```python
from build123d import *

# Parameters (mm, degrees)
SKETCH_1_W      = 200
SKETCH_1_H      = 200
SKETCH_1_R      = 5
EXTRUDE_1_DEPTH = 5
CHAMFER_1_SIZE  = 3


with BuildPart() as part:
    # Эскиз1 → Бобышка-Вытянуть1 (new body)
    with BuildSketch(Plane(origin=(0, 0, 0), x_dir=(1, 0, 0), z_dir=(0, 1, 0))):
        Rectangle(SKETCH_1_W, SKETCH_1_H)
        Circle(SKETCH_1_R, mode=Mode.SUBTRACT)
    extrude(amount=EXTRUDE_1_DEPTH)

    # Фаска1
    chamfer_1_edges = [part.edges().sort_by_distance(p)[0] for p in [
        (-5, 0, 0),
    ]]
    chamfer(chamfer_1_edges, length=CHAMFER_1_SIZE)


solid = part.part
```
Input: part model. Units: mm. Frame: model coordinates. Coordinates: 2 decimals unless noted, no trailing zeros. Loops run counter-clockwise (first coordinate to the right, second up) from the corner with the lowest first, then second, coordinate; pieces in that order, holes last. Notation, with made-up numbers: (70, -12) - (108, -12) arc R30 cw to (108, 15) - close; hole circle Ø2 at (-30.5, 3.5). An arc over 180 degrees is marked (long way). Answer in a Markdown table with one row per item.
(1) Mould query, pull axis X, two halves, no side actions, for faces 1 (the face through (4.95, 2.81, -1.56)), 2 (the face through (-1, 0, -24)), 3 (the face through (100, 2, 1)). Classes: pulls with the +X half, pulls with the -X half, needs draft (parallel to the pull), parting line crosses it, or undercut.
Model answer:
| item | result |
|---|---|
| face 1 | undercut |
| face 2 | needs draft |
| face 3 | pulls with the +X half |
(2) Material intervals for L1, parallel to X at y = 4.45, z = 0, sorted ascending. Write a range as from..to.
Model answer:
| item | result |
|---|---|
| L1 | x = -100..-5, 5..100 |
(3) Cut plane B-B on z = 0. Output: boundary loops of the cut face in (x, y).
Model answer:
| item | result |
|---|---|
| outline | (-100, 0) - (-8, 0) - (-5, 3) - (-5, 5) - (-100, 5) - close; (5, 3) - (8, 0) - (100, 0) - (100, 5) - (5, 5) - close |
(4) Cut plane A-A on x = 0. Output: boundary loops of the cut face in (y, z).
Model answer:
| item | result |
|---|---|
| outline | (0, -100) - (5, -100) - (5, -5) - (3, -5) - (0, -8) - close; (0, 8) - (3, 5) - (5, 5) - (5, 100) - (0, 100) - close |
(5) Pin query (flat end, axial travel): P1, Ø9, axis at x = 0, z = 0, coming from the +Y side; P2, Ø1.5, axis at x = 59, z = 57.5, coming from the -Y side. Return the tip coordinate at first contact, or that it passes through.
Model answer:
| item | result |
|---|---|
| P1 | passes through |
| P2 | stops at y = 0 |
